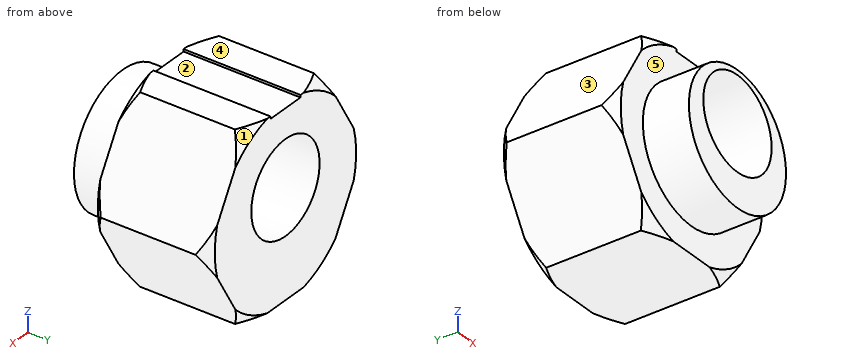
from build123d import *

# Parameters (mm, degrees)
BOSS_EXTRUDE1_DEPTH = 6.35
SKETCH3_R           = 3.555
BOSS_EXTRUDE3_DEPTH = 2.5
SKETCH4_R           = 2.5
CUT_EXTRUDE1_DEPTH  = 9.85
SKETCH5_W           = 2.2
SKETCH5_H           = 0.13
CUT_EXTRUDE2_DEPTH  = 7.35


with BuildPart() as part:
    # Sketch1 → Boss-Extrude1 (new body)
    with BuildSketch(Plane(origin=(0, 0, 0), x_dir=(1, 0, 0), z_dir=(0, 1, 0))):
        Polygon((5.773502692, 0), (2.886751346, 5), (-2.886751346, 5), (-5.773502692, 0), (-2.886751346, -5), (2.886751346, -5), align=None)
    extrude(amount=BOSS_EXTRUDE1_DEPTH)

    # Sketch3 → Boss-Extrude3 (add)
    with BuildSketch(Plane.XZ):
        Circle(SKETCH3_R)
    extrude(amount=BOSS_EXTRUDE3_DEPTH)

    # Sketch4 → Cut-Extrude1 (cut, through all)
    with BuildSketch(Plane(origin=(0, 6.35, 0), x_dir=(1, 0, 0), z_dir=(0, 1, 0))):
        with Locations((0, -0.79)):
            Circle(SKETCH4_R)
    extrude(amount=-CUT_EXTRUDE1_DEPTH, mode=Mode.SUBTRACT)

    # Sketch5 → Cut-Extrude2 (cut, through all)
    with BuildSketch(Plane(origin=(0, 0, 0), x_dir=(-1, 0, 0), z_dir=(0, -1, 0))):
        with Locations((0, -4.935)):
            Rectangle(SKETCH5_W, SKETCH5_H)
    extrude(amount=-CUT_EXTRUDE2_DEPTH, mode=Mode.SUBTRACT)

    # Sketch6 → Cut-Revolve1 (revolve, cut)
    with BuildSketch(Plane.XY):
        Polygon((5.173502692, 6.35), (5.773502692, 6.35), (5.773502692, 5.75), align=None)
        Polygon((5.773502692, 0.6), (5.173502692, 0), (5.773502692, 0), align=None)
    revolve(axis=Axis((0, 0, 0), (0, 1, 0)), mode=Mode.SUBTRACT)


solid = part.part
Source: CAD feature listing. Evaluate the final solid. Frame: model axes, mm. Face numbers are marked on the shaded views. A direction names the side the tool comes from. Round coordinates to 2 decimals unless told otherwise and drop trailing zeros. Loops run counter-clockwise (first coordinate to the right, second up) from the corner with the lowest first, then second, coordinate; pieces in that order, holes last. Notation, with made-up numbers: M 4.5,29 L 24.5,29 A5 cw 24.5,35 Z; hole C 61,78.5 d5. An arc over 180 degrees is marked long. Return JSON: item names as keys, results as strings. Group by question number.
1. Material intervals for line 1 along Z through (x, y) = (0, -0.5) (3 decimals); line 2 along Z through (x, y) = (0, 2); line 3 along Y through (x, z) = (3.25, -2), sorted ascending. Write a range as from..to.
2. Section query B-B on y = 3.25. Output: boundary loops of the cut face in (x, z), and give its area (3 significant figures).
3. Reachability of the marked faces 4 and 5 from +Z, -Z, +X, -X, +Y, -Y: full face, straight path, thin tool, end or side. Return the list, or none.
4. Section query C-C on z = 2.5. Output: boundary loops of the cut face in (x, y), and give its area (3 significant figures).
5. Mould query, pull axis X, two halves, no side actions, for the marked faces 1, 2 and 3. Classes: released by +X, released by -X, zero draft, split by the parting line, or undercut.
6. Pin query (flat end, axial travel): pin 1 (1.5 mm diameter, centred on x = -0.5, z = 3, fed in from -Y); pin 2 (4 mm diameter, centred on y = 1, z = -2.5, fed in from +X); pin 3 (2 mm diameter, centred on y = 3.5, z = -1.5, fed in from -X). Return the tip coordinate at first contact, or that it passes through.
7. Section query A-A on x = 0. Output: boundary loops of the cut face in (y, z) (3 decimals).
8. Section query D-D on z = -2. Output: boundary loops of the cut face in (x, y).
Checks:
{
 "1": {"line 1": "z = -3.555..-1.71, 3.29..3.555", "line 2": "z = -5..-1.71, 3.29..4.87", "line 3": "y = 0..6.35"},
 "2": {"outline": "M -5.77,0 L -2.89,-5 L 2.89,-5 L 5.77,0 L 2.89,5 L 1.1,5 L 1.1,4.87 L -1.1,4.87 L -1.1,5 L -2.89,5 Z; hole C 0,0.79 d5", "area": "66.7 mm²"},
 "3": {"face 4": "+Z, +X, -X, +Y, -Y", "face 5": "-Y"},
 "4": {"outline": "M -4.33,0 L -2.53,0 L -2.53,-2.5 L -1.82,-2.5 L -1.82,6.35 L -4.33,6.35 Z; M 1.82,-2.5 L 2.53,-2.5 L 2.53,0 L 4.33,0 L 4.33,6.35 L 1.82,6.35 Z", "area": "35.4 mm²"},
 "5": {"face 1": "released by +X", "face 2": "undercut", "face 3": "released by -X"},
 "6": {"pin 1": "stops at y = -2.5", "pin 2": "stops at x = 5.48", "pin 3": "stops at x = -5.48"},
 "7": {"outline": "M -2.5,-3.555 L 0,-3.555 L 0,-5 L 6.35,-5 L 6.35,-1.71 L -2.5,-1.71 Z; M -2.5,3.29 L 6.35,3.29 L 6.35,4.87 L 0,4.87 L 0,3.555 L -2.5,3.555 Z"},
 "8": {"outline": "M -4.62,0 L -2.94,0 L -2.94,-2.5 L 2.94,-2.5 L 2.94,0 L 4.62,0 L 4.62,6.35 L -4.62,6.35 Z"}
}
